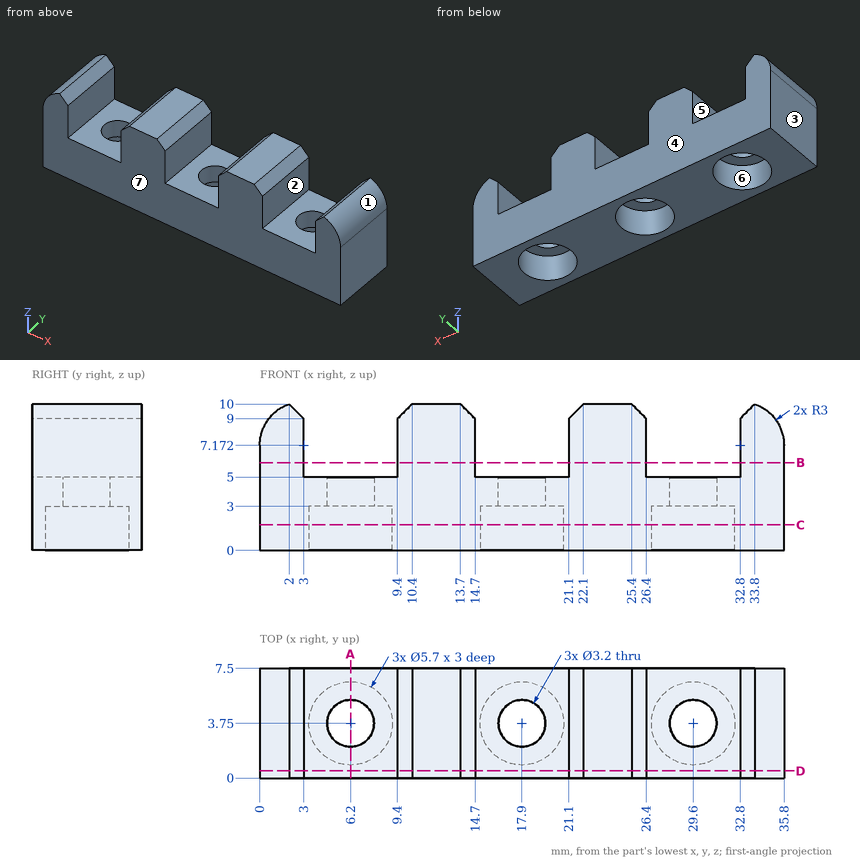
Could you check a few things on this drawing? It's one solid part, dimensions in mm from its lowest x, y, z. A direction names the side the tool comes from. Give positions to 0.01 mm unless a question says otherwise; leave off trailing zeros. Loops run counter-clockwise (first coordinate to the right, second up) from the corner with the lowest first, then second, coordinate; pieces in that order, holes last. Notation, with made-up numbers: (52.25, 74.5) -> (96.25, 74.5) arc R31 ccw to (96.25, 105.5) -> close; hole circle Ø11 at (-23, 88). An arc over 180 degrees is marked (long way). Answer as CSV lines item,"result". Start each with the question number.
(1) We'd pull the mould along X, two halves only. Please class the marked faces 1, 2, 3 and 4: released by +X, released by -X, zero draft, split by the parting line, or undercut.
(2) If we section it at D-D on y = 0.5: Write out the boundary of the cut face in (x, z).
(3) Which directions (+Z, -Z, +X, -X, +Y, -Y) give clear straight access to the entire face, cutting with the end or side of a thin tool? Please do the marked faces 5, 6 and 7.
(4) I need wall thicknesses on probe 1 along X at (y, z) = (6, 5.25); probe 2 along Y at (x, z) = (17.9, 4.5); probe 3 along Y at (x, z) = (6.2, 1.95). Which ranges of each line are inside material? Lowest first, please.
(5) If we section it at C-C on z = 1.75: Write out the boundary of the cut face in (x, y), then the cut area to 3 significant figures.
(6) I'm going to push flat-ended pins straight in: pin 1 Ø4.5 at (x, y) = (29.6, 3.75) entering from +Z; pin 2 Ø1.5 at (y, z) = (4, 8) entering from -X. Where does each tip first touch, or does it pass through?
(7) If we section it at A-A on x = 6.2: Write out the boundary of the cut face in (y, z).
(8) If we section it at B-B on z = 6: Write out the boundary of the cut face in (x, y).
Computed:
1,face 1,"released by +X"
1,face 2,"undercut"
1,face 3,"released by -X"
1,face 4,"zero draft"
2,outline,"(0, 0) -> (35.8, 0) -> (35.8, 7.17) arc R3 ccw to (33.8, 10) -> (32.8, 9) -> (32.8, 5) -> (26.4, 5) -> (26.4, 9) -> (25.4, 10) -> (22.1, 10) -> (21.1, 9) -> (21.1, 5) -> (14.7, 5) -> (14.7, 9) -> (13.7, 10) -> (10.4, 10) -> (9.4, 9) -> (9.4, 5) -> (3, 5) -> (3, 9) -> (2, 10) arc R3 ccw to (0, 7.17) -> close"
3,face 5,"+Z, +Y, -Y"
3,face 6,"-Z"
3,face 7,"+Z, -Z, +X, -X, -Y"
4,probe 1,"x = 0 to 3, 9.4 to 14.7, 21.1 to 26.4, 32.8 to 35.8"
4,probe 2,"y = 0 to 2.15, 5.35 to 7.5"
4,probe 3,"y = 0 to 0.9, 6.6 to 7.5"
5,outline,"(0, 0) -> (35.8, 0) -> (35.8, 7.5) -> (0, 7.5) -> close; hole circle Ø5.7 at (6.2, 3.75); hole circle Ø5.7 at (17.9, 3.75); hole circle Ø5.7 at (29.6, 3.75)"
5,area,"192 mm2"
6,pin 1,"stops at z = 5"
6,pin 2,"stops at x = 0"
7,outline,"(0, 0) -> (0.9, 0) -> (0.9, 3) -> (2.15, 3) -> (2.15, 5) -> (0, 5) -> close; (5.35, 3) -> (6.6, 3) -> (6.6, 0) -> (7.5, 0) -> (7.5, 5) -> (5.35, 5) -> close"
8,outline,"(0, 0) -> (3, 0) -> (3, 7.5) -> (0, 7.5) -> close; (9.4, 0) -> (14.7, 0) -> (14.7, 7.5) -> (9.4, 7.5) -> close; (21.1, 0) -> (26.4, 0) -> (26.4, 7.5) -> (21.1, 7.5) -> close; (32.8, 0) -> (35.8, 0) -> (35.8, 7.5) -> (32.8, 7.5) -> close"
